Could you check a few things on this model? Use its own coordinates, in mm. Give positions to 0.01 mm unless a question says otherwise; leave off trailing zeros. Write each loop counter-clockwise with the first axis right and the second up, starting at its lowest first coordinate (ties: lowest second). Pieces come first, ordered by that corner, then holes. Notation, with made-up numbers: M -10.75,6 L 16.25,6 A14 ccw 16.25,32 Z; hole C 85.5,-12.5 d4. An arc over 180 degrees is marked long. Use one line per item in the form item = value.
from build123d import *

# Parameters (mm, degrees)
F0_R      = 35
F1_DEPTH  = 100
F1_FACE_R = 35
F2_DEPTH  = 90
F2_TAPER  = 12
F3_DEPTH  = 10


with BuildPart() as f1:
    # F0 (on Top) → F1 (new body)
    with BuildSketch(Plane.XY):
        Circle(F0_R)
    extrude(amount=F1_DEPTH)

    # F1_face (on face) → F2 (join)
    with BuildSketch(Plane.XY.offset(100)):
        Circle(F1_FACE_R)
    extrude(amount=F2_DEPTH, taper=F2_TAPER)

    # F3 (add): a face of the model
    f3_faces = [f1.faces().sort_by_distance(p)[0] for p in [
        (0, 0, 190),
    ]]
    extrude(f3_faces, amount=F3_DEPTH)


solid = f1.part
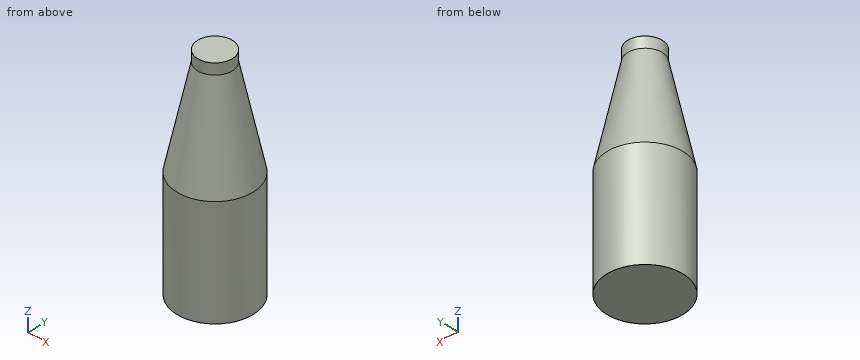
1) If I drill on L1, parallel to X at y = -1, z = 85; L2, parallel to Y at x = -17.5, z = 33; L3, parallel to Y at x = 12, z = 133.5, over which ranges is the centre line in solid material (lowest first)?
Checked values:
L1 = -34.99 to 34.99
L2 = -30.31 to 30.31
L3 = -25.16 to 25.16
2) I want a section at C-C, the plane z = 60.5. Please give me the cut outline in (x, y).
Checked values:
outline = C 0,0 d70
3) I want a section at D-D, the plane z = 137.5. Please give me the cut outline in (x, y).
Checked values:
outline = C 0,0 d54.06
4) For pin 1 Ø4 at (x, z) = (18, 161) entering from +Y; pin 2 Ø1 at (y, z) = (-12.5, 114) entering from -X; pin 3 Ø2 at (x, z) = (0, 87.5) entering from +Y, each with a flat end and sliding along its axis, tell me the tip position at first contact or that it passes through.
Checked values:
pin_1 = 15.24
pin_2 = -29.72
pin_3 = 35
5) I want a section at A-A, the plane x = 0. Please give me the cut outline in (y, z), plus the area to 3 significant figures.
Checked values:
outline = M -35,0 L 35,0 L 35,100 L 15.87,190 L 15.87,200 L -15.87,200 L -15.87,190 L -35,100 Z
area = 11,900 mm2
